CAD build for the part. Positions are in the model's coordinates, mm. Face numbers are marked on the shaded views. A direction names the side the tool comes from. Round coordinates to 2 decimals unless told otherwise and drop trailing zeros. Order: outer loops, then holes, each group sorted by start corner. A loop starts at its lowest first (then second) coordinate and runs counter-clockwise, first axis right, second up. Notation, with made-up numbers: (-12.5, -12.75) - (21.5, -12.75) arc R19 cw to (21.5, 12.25) - close; hole circle Ø3 at (26.5, 49.5). An arc over 180 degrees is marked (long way). Use one line per item in the form item = value. Start each with the question number.
Autodesk Inventor part; units mm, degrees
ref_plane "YZ Plane" through (0, 0, 0) normal (1, 0, 0) x (0, 1, 0)
ref_plane "XZ Plane" through (0, 0, 0) normal (0, 1, 0) x (-1, 0, 0)
ref_plane "XY Plane" through (0, 0, 0) normal (0, 0, 1) x (1, 0, 0)
sketch "Sketch1" plane through (0, 0, 0) normal (0, 1, 0) x (-1, 0, 0)
  circle A0 centre (0, 0) radius 8
  dimension "d0" = 16
extrude "Extrusion1" add sketch "Sketch1" along normal blind 20
sketch "Sketch2" plane through (0, 20, 0) normal (0, 1, 0) x (1, 0, 0)
  circle A0 centre (0, 0) radius 9.5
  dimension "d3" = 19
extrude "Extrusion2" add sketch "Sketch2" along normal blind 2.5
chamfer "Chamfer1" distance 2 angle 45 1 edges at (-9.5, 22.5, 0)
sketch "Sketch3" plane through (0, 22.5, 0) normal (0, 1, 0) x (1, 0, 0)
  circle A0 centre (0, 0) radius 5.5
  circle A1 centre (0, 0) radius 6.75
  dimension "d9" = 11
  dimension "d10" = 13.5
extrude "Extrusion3" cut sketch "Sketch3" against normal blind 0.1
properties part number "16mm_switch"
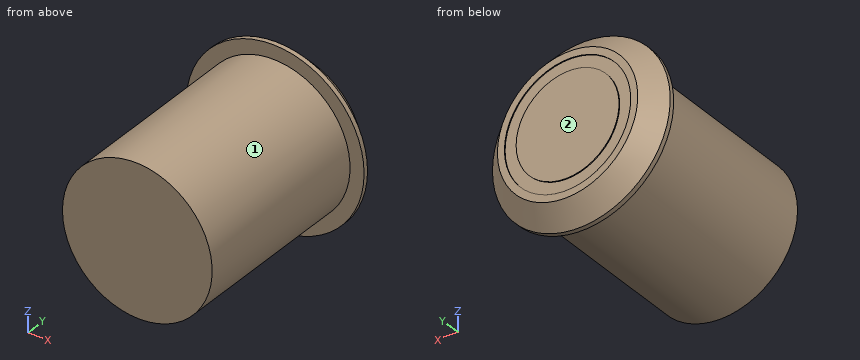
(1) Slice it at A-A (z = 0). Give the cut face in (x, y).
(2) Wall check: line 1 (Z direction, x = 0.25, y = 6); line 2 (Y direction, x = 1.75, z = -5.5); line 3 (Z direction, x = 0, y = 22.45). Give the ranges that are in metal, low to high. Write a range as [from, to].
(3) Slice it at B-B (x = 0). Give the cut face in (y, z).
(4) Flat gauge pins, fed straight in: P1, Ø3, axis at x = 0, y = 15, coming from the +Z side; P2, Ø4, axis at x = -6.5, y = 19.5, coming from the +Z side; P3, Ø6, axis at y = 9.5, z = 6, coming from the +X side. Where does each tip first touch, or does it go through?
(5) Which spindle directions (+Z, -Z, +X, -X, +Y, -Y) get a long thin tool onto all of the face, cutting with end or side? Do the marked faces 1 and 2. Say none if no direction does.
(6) Slice it at C-C (y = 9.5). Give the cut face in (x, z).
Results list:
q1.outline = (-9.5, 20) - (-8, 20) - (-8, 0) - (8, 0) - (8, 20) - (9.5, 20) - (9.5, 20.5) - (7.5, 22.5) - (6.75, 22.5) - (6.75, 22.4) - (5.5, 22.4) - (5.5, 22.5) - (-5.5, 22.5) - (-5.5, 22.4) - (-6.75, 22.4) - (-6.75, 22.5) - (-7.5, 22.5) - (-9.5, 20.5) - close
q2.line_1 = [-8, 8]
q2.line_2 = [0, 22.4]
q2.line_3 = [-7.55, -6.75], [-5.5, 5.5], [6.75, 7.55]
q3.outline = (0, -8) - (20, -8) - (20, -9.5) - (20.5, -9.5) - (22.5, -7.5) - (22.5, -6.75) - (22.4, -6.75) - (22.4, -5.5) - (22.5, -5.5) - (22.5, 5.5) - (22.4, 5.5) - (22.4, 6.75) - (22.5, 6.75) - (22.5, 7.5) - (20.5, 9.5) - (20, 9.5) - (20, 8) - (0, 8) - close
q4.P1 = 8
q4.P2 = 8.33
q4.P3 = 7.42
q5.face_1 = -Y
q5.face_2 = +Z, -Z, +X, -X, +Y
q6.outline = circle Ø16 at (0, 0)
